from build123d import *

# Parameters (mm, degrees)
SKETCH_1_R          = 8
EXTRUDE_1_DEPTH     = 10
CUT_EXTRUDE_2_DEPTH = 3
CUT_EXTRUDE_3_DEPTH = 3
FILLET_1_R          = 2


with BuildPart() as part:
    # 草图1 → 凸台-拉伸1 (new body)
    with BuildSketch(Plane.XY):
        with BuildLine():
            Line((-56.424978154, 18.5), (-56.424978154, 0))
            Line((-56.424978154, 0), (-36.424978154, 0))
            Line((-36.424978154, 0), (-12.510711799, 10.595719206))
            Line((-12.510711799, 10.595719206), (-12.510711799, 13.595719206))
            Line((-12.510711799, 13.595719206), (7.489288201, 13.595719206))
            Line((7.489288201, 13.595719206), (13.872204282, 0))
            Line((13.872204282, 0), (74.552459824, 0))
            Line((74.552459824, 0), (78.025423377, 19.69615506))
            Line((78.025423377, 19.69615506), (123.025423377, 19.69615506))
            Line((123.025423377, 19.69615506), (123.025423377, 54.69615506))
            Line((123.025423377, 54.69615506), (58.025423377, 54.69615506))
            add(Edge.make_bspline(
                [(58.025423377, 54.69615506), (48.897941568, 54.692205697), (43.17687282, 53.988854745), (35.233696766, 52.670853795)],
                knots=[0, 0, 0, 0, 1, 1, 1, 1], degree=3))
            Line((35.233696766, 52.670853795), (35.233696766, 49.670853795))
            add(Edge.make_bspline(
                [(35.233696766, 49.670853795), (10.57425282, 44.720207412), (-12.510711799, 32.467844976)],
                knots=[0, 0, 0, 1, 1, 1], degree=2))
            Line((-12.510711799, 32.467844976), (-12.510711799, 35.467844976))
            Line((-12.510711799, 35.467844976), (-56.424978154, 18.5))
        make_face()
        with Locations((45.747275879, 36.3493933)):
            Circle(SKETCH_1_R, mode=Mode.SUBTRACT)
    extrude(amount=EXTRUDE_1_DEPTH)

    # 草图2 → 切除-拉伸2 (cut)
    with BuildSketch(Plane.XY.offset(10)):
        with BuildLine():
            Line((-12.510711799, 32.467844976), (-12.510711799, 13.595719206))
            Line((-12.510711799, 13.595719206), (7.489288201, 13.595719206))
            Line((7.489288201, 13.595719206), (13.872204282, 0))
            Line((13.872204282, 0), (74.552459824, 0))
            Line((74.552459824, 0), (78.025423377, 19.69615506))
            Line((78.025423377, 19.69615506), (123.025423377, 19.69615506))
            Line((123.025423377, 19.69615506), (123.025423377, 33.69615506))
            Line((123.025423377, 33.69615506), (78.025423377, 33.69615506))
            add(Edge.make_bspline(
                [(69.768901699, 40.433897673), (72.258439371, 38.402308014), (75.204387373, 35.998264258), (78.025423377, 33.69615506)],
                knots=[0, 0, 0, 0, 1, 1, 1, 1], degree=3))
            add(Edge.make_bspline(
                [(35.233696766, 46.670853795), (56.25429865, 47.512975461), (69.768901699, 40.433897673)],
                knots=[0, 0, 0, 1, 1, 1], degree=2))
            Line((35.233696766, 46.670853795), (35.233696766, 49.670853795))
            add(Edge.make_bspline(
                [(-12.510711799, 32.467844976), (10.107568712, 45.643152542), (35.233696766, 49.670853795)],
                knots=[0, 0, 0, 1, 1, 1], degree=2))
        make_face()
    extrude(amount=-CUT_EXTRUDE_2_DEPTH, mode=Mode.SUBTRACT)

    # 草图3 → 切除-拉伸3 (cut)
    with BuildSketch(Plane(origin=(0, 0, 0), x_dir=(-1, 0, 0), z_dir=(0, 0, -1))):
        with BuildLine():
            Line((-123.025423377, 19.69615506), (-78.025423377, 19.69615506))
            Line((-78.025423377, 19.69615506), (-74.552459824, 0))
            Line((-74.552459824, 0), (-13.872204282, 0))
            Line((-13.872204282, 0), (-7.489288201, 13.595719206))
            Line((-7.489288201, 13.595719206), (12.510711799, 13.595719206))
            Line((12.510711799, 13.595719206), (12.510711799, 32.467844976))
            add(Edge.make_bspline(
                [(-35.233696766, 49.670853795), (-9.646215757, 44.931714493), (12.510711799, 32.467844976)],
                knots=[0, 0, 0, 1, 1, 1], degree=2))
            Line((-35.233696766, 49.670853795), (-35.233696766, 46.670322435))
            add(Edge.make_bspline(
                [(-35.233696766, 46.670322435), (-53.573988888, 48.036148069), (-69.589003354, 41.428180454)],
                knots=[0, 0, 0, 1, 1, 1], degree=2))
            add(Edge.make_bspline(
                [(-69.589003354, 41.428180454), (-74.339147925, 38.238278194), (-78.025423377, 33.69615506)],
                knots=[0, 0, 0, 1, 1, 1], degree=2))
            Line((-78.025423377, 33.69615506), (-123.025423377, 33.69615506))
            Line((-123.025423377, 33.69615506), (-123.025423377, 19.69615506))
        make_face()
    extrude(amount=-CUT_EXTRUDE_3_DEPTH, mode=Mode.SUBTRACT)

    # 圆角1
    fillet_1_edges = [part.edges().sort_by_distance(p)[0] for p in [
        (-12.510711799, 10.595719206, 5),
        (-36.424978154, 0, 5),
        (-56.424978154, 0, 5),
        (-56.424978154, 18.5, 5),
        (123.025423377, 19.69615506, 5),
        (78.025423377, 19.69615506, 5),
        (74.552459824, 0, 5),
        (13.872204282, 0, 5),
        (7.489288201, 13.595719206, 5),
    ]]
    fillet(fillet_1_edges, radius=FILLET_1_R)


solid = part.part
Design review of the part built by this model. Coordinates are the model's own, in mm. A direction names the side the tool comes from. Coordinates: 2 decimals unless noted, no trailing zeros. Order: outer loops, then holes, each group sorted by start corner. A loop starts at its lowest first (then second) coordinate and runs counter-clockwise, first axis right, second up.
Item 1: For line 1 (Z direction, x = 31, y = 30); line 2 (Z direction, x = 69.5, y = 41); line 3 (Y direction, x = 110, z = 0.5), list the stretches that pass through material, from the lowest coordinate up.
Item 2: For pin 1 Ø25 at (x, y) = (68.5, 27.5) entering from +Z; pin 2 Ø3 at (x, z) = (92.5, 4) entering from -Y; pin 3 Ø1 at (y, z) = (28, 2) entering from +X; pin 4 Ø3 at (x, y) = (-0.5, 21.5) entering from -Z, all flat-tipped, find the tip position at first contact; note any pin that passes through.
Item 3: For faces 1 (the flat face through (-3, 13.596, 5)), 2 (the flat face through (101, 33.696, 9)), 3 (the flat face through (35.234, 50, 5)), 4 (the flat face through (100, 19.696, 5)), list the 3-axis set-ups (+Z, -Z, +X, -X, +Y, -Y) from which the entire face can be reached by the end or side of a thin tool; tool diameter is ignored.
Item 4: Take a section at B-B, the plane x = -41. Write out the cut boundary in (y, z).
Item 5: Take a section at A-A, the plane y = 5. Write out the cut boundary in (x, z), then the cut area to 3 significant figures.
Item 6: The part is to be moulded in two halves that separate along X. For faces 5 (the flat face through (-35, 14, 0)), 6 (the flat face through (10.64, 6.88, 4.97)), 7 (the flat face through (76.27, 9.73, 4.97)), say which applies: pulls with the +X half, pulls with the -X half, needs draft (parallel to the pull), parting line crosses it, or undercut.
The answers:
1. line 1: z = 3 to 7
1. line 2: z = 3 to 10
1. line 3: y = 33.7 to 54.7
2. pin 1: stops at z = 10
2. pin 2: stops at y = 19.7
2. pin 3: stops at x = -12.51
2. pin 4: stops at z = 3
3. face 1: +Z, -Z, -Y
3. face 2: +Z, +X, -Y
3. face 3: -X, +Y
3. face 4: +Z, -Z, +X, -Y
4. outline: (0, 0) - (24.46, 0) - (24.46, 10) - (0, 10) - close
5. outline: (-56.42, 0) - (-25.14, 0) - (-25.14, 10) - (-56.42, 10) - close; (11.52, 3) - (75.43, 3) - (75.43, 7) - (11.52, 7) - close
5. area: 568 mm2
6. face 5: needs draft
6. face 6: undercut
6. face 7: pulls with the +X half
